Autodesk Inventor part; units mm, degrees
ref_plane "YZ Plane" through (0, 0, 0) normal (1, 0, 0) x (0, 1, 0)
ref_plane "XZ Plane" through (0, 0, 0) normal (0, 1, 0) x (-1, 0, 0)
ref_plane "XY Plane" through (0, 0, 0) normal (0, 0, 1) x (1, 0, 0)
sketch "Sketch1" plane through (0, 0, 0) normal (0, 1, 0) x (-1, 0, 0)
  line L0 (0, 0) -> (711.2, 0)
  line L1 (711.2, 0) -> (711.2, -812.8)
  line L2 (711.2, -812.8) -> (0, -812.8)
  line L3 (0, -812.8) -> (0, 0)
  line L4 (0, 0) -> (711.2, 0)
  line L5 (711.2, 0) -> (711.2, -76.2)
  line L6 (0, -76.2) -> (0, 0)
  line L7 (0, -812.8) -> (711.2, -812.8)
  line L8 (711.2, -812.8) -> (711.2, -736.6)
  line L9 (0, -736.6) -> (0, -812.8)
  line L10 (0, 0) -> (25.4, 0)
  line L11 (25.4, -76.2) -> (25.4, -736.6)
  line L12 (25.4, -812.8) -> (0, -812.8)
  line L13 (0, -812.8) -> (0, 0)
  line L14 (711.2, 0) -> (685.8, 0)
  line L15 (685.8, -76.2) -> (685.8, -736.6)
  line L16 (685.8, -812.8) -> (711.2, -812.8)
  line L17 (711.2, -812.8) -> (711.2, 0)
  line L18 (685.8, -736.6) -> (635, -736.6)
  line L19 (615.95, -736.6) -> (615.95, -76.2)
  line L20 (635, -76.2) -> (635, -736.6)
  line L21 (25.4, -736.6) -> (76.2, -736.6)
  line L22 (95.25, -736.6) -> (95.25, -76.2)
  line L23 (76.2, -76.2) -> (76.2, -736.6)
  line L24 (685.8, -76.2) -> (635, -76.2)
  line L25 (685.8, -736.6) -> (635, -736.6)
  line L26 (615.95, -736.6) -> (95.25, -736.6)
  line L27 (76.2, -736.6) -> (25.4, -736.6)
  line L28 (615.95, -76.2) -> (95.25, -76.2)
  line L29 (76.2, -76.2) -> (25.4, -76.2)
  dimension "d0" = 711.2
  dimension "d1" = 812.8
  dimension "d2" = 76.2
  dimension "d3" = 76.2
  dimension "d4" = 25.4
  dimension "d5" = 25.4
  dimension "d6" = 812.8
  dimension "d10" = 660.4
extrude "Extrusion1" add sketch "Sketch1" along normal blind 3.175
sketch "Sketch2" plane through (0, 3.175, 0) normal (0, 1, 0) x (1, 0, 0)
  line L0 (-711.2, 812.8) -> (0, 812.8)
  line L1 (0, 812.8) -> (0, 0)
  line L2 (0, 0) -> (-711.2, 0)
  line L3 (-711.2, 0) -> (-711.2, 812.8)
  line L4 (-708.025, 809.625) -> (-3.175, 809.625)
  line L5 (-3.175, 809.625) -> (-3.175, 3.175)
  line L6 (-3.175, 3.175) -> (-708.025, 3.175)
  line L7 (-708.025, 3.175) -> (-708.025, 809.625)
extrude "Extrusion2" add sketch "Sketch2" along normal blind 73.025
sketch "Sketch3" plane through (0, 0, 0) normal (0, -1, 0) x (1, 0, 0)
  line L0 (-25.4, -76.2) -> (-25.4, -50.8)
  line L1 (-25.4, -50.8) -> (-685.8, -50.8)
  line L2 (-685.8, -50.8) -> (-685.8, -762)
  line L3 (-685.8, -762) -> (-25.4, -762)
  line L4 (-25.4, -762) -> (-25.4, -50.8)
  line L5 (-25.4, -76.2) -> (-76.2, -76.2)
  line L6 (-76.2, -76.2) -> (-76.2, -50.8)
  line L7 (-95.25, -76.2) -> (-95.25, -50.8)
  line L8 (-95.25, -76.2) -> (-615.95, -76.2)
  line L9 (-615.95, -76.2) -> (-615.95, -50.8)
  line L10 (-635, -76.2) -> (-635, -50.8)
  line L11 (-635, -76.2) -> (-685.8, -76.2)
  line L12 (-95.25, -736.6) -> (-95.25, -762)
  line L13 (-95.25, -736.6) -> (-615.95, -736.6)
  line L14 (-615.95, -736.6) -> (-615.95, -762)
  line L15 (-635, -736.6) -> (-635, -762)
  line L16 (-635, -736.6) -> (-685.8, -736.6)
  line L17 (-635, -50.8) -> (-685.8, -50.8)
  line L18 (-685.8, -50.8) -> (-685.8, -76.2)
  line L19 (-685.8, -736.6) -> (-685.8, -762)
  line L20 (-685.8, -762) -> (-635, -762)
  line L21 (-615.95, -762) -> (-95.25, -762)
  line L22 (-95.25, -762) -> (-95.25, -736.6)
  line L23 (-25.4, -736.6) -> (-25.4, -76.2)
  line L24 (-25.4, -762) -> (-76.2, -762)
  line L25 (-76.2, -762) -> (-76.2, -736.6)
  line L26 (-76.2, -736.6) -> (-25.4, -736.6)
  line L27 (-25.4, -736.6) -> (-25.4, -762)
  point P0 (0, 0)
  dimension "d22" = 25.4
  dimension "d23" = 660.4
  dimension "d24" = 711.2
  dimension "d25" = 25.4
  dimension "d26" = 25.4
extrude "Extrusion3" cut sketch "Sketch3" against normal blind 73.025 contours L5 L6 L1 L0 | L4 L3 L25 L26 | L7 L8 L9 L1 | L3 L14 L13 L12 | L10 L11 L2 L1 | L3 L2 L16 L15
sketch "Sketch4" plane through (-711.2, 0, -812.8) normal (-1, 0, 0) x (0, 0, 1)
  line L0 (812.8, 76.2) -> (406.4, 76.2)
  line L1 (812.8, 76.2) -> (0, 76.2)
  line L2 (762, 0) -> (50.8, 0)
  circle A0 centre (406.4, 63.5) radius 6.35
  circle A1 centre (711.2, 63.5) radius 6.35
  circle A2 centre (101.6, 63.5) radius 6.35
  point P0 (812.8, 0)
  dimension "d29" = 406.4
  dimension "d31" = 12.7
  dimension "d35" = 12.7
  dimension "d36" = 12.7
sketch "Sketch5" plane through (0, 3.175, 0) normal (0, 1, 0) x (1, 0, 0)
  line L0 (-708.025, 3.175) -> (-3.175, 3.175)
  line L1 (-3.175, 809.625) -> (-708.025, 809.625)
  line L2 (-615.95, 3.175) -> (-619.125, 3.175)
  line L3 (-619.125, 3.175) -> (-619.125, 809.625)
  line L4 (-619.125, 809.625) -> (-615.95, 809.625)
  line L5 (-615.95, 809.625) -> (-615.95, 3.175)
  line L6 (-95.25, 809.625) -> (-92.075, 809.625)
  line L7 (-92.075, 809.625) -> (-92.075, 3.175)
  line L8 (-92.075, 3.175) -> (-95.25, 3.175)
  line L9 (-95.25, 3.175) -> (-95.25, 809.625)
  point P0 (0, 0)
  dimension "d37" = 3.175
  dimension "d38" = 3.175
extrude "Extrusion4" add sketch "Sketch5" along normal blind 73.025 contours L3 L1 L5 L0 | L9 L1 L7 L0
extrude "Extrusion5" cut sketch "Sketch4" against normal blind 1016
properties part number "Base"
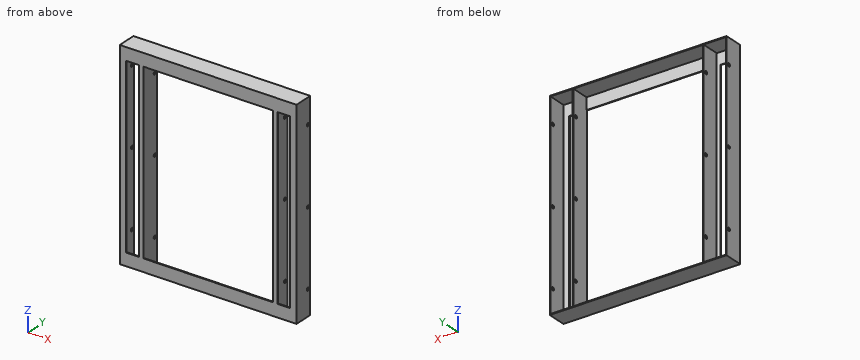
The model under review builds one solid part; all positions refer to its coordinate system, in mm. Round coordinates to 2 decimals unless told otherwise and drop trailing zeros. Write each loop counter-clockwise with the first axis right and the second up, starting at its lowest first coordinate (ties: lowest second). Pieces come first, ordered by that corner, then holes. Notation, with made-up numbers: (-34, 50) - (-1, 50) arc R17 cw to (-1, 73) - close; hole circle Ø7 at (3, -9.5). An arc over 180 degrees is marked (long way). One line per item, written item: value. Start each with the question number.
1. To check wall thickness, follow L1, parallel to X at y = 58, z = -57 (3 decimals); L2, parallel to X at y = 3, z = -294; L3, parallel to Y at x = -94.1, z = -406.4. State the ranges of each line that lie inside material, in increasing order. Write a range as from..to.
2. Consider section A-A on x = -214. Write out the cut boundary in (y, z) (3 decimals), and give its area (3 significant figures).
3. Consider section B-B on z = -142. Write out the cut boundary in (x, y) (3 decimals), and give its area (3 significant figures).
Checks:
1. L1: x = -711.2..-708.025, -619.125..-615.95, -95.25..-92.075, -3.175..0
1. L2: x = -711.2..-685.8, -635..-615.95, -95.25..-76.2, -25.4..0
1. L3: y = 0..57.15, 69.85..76.2
2. outline: (0, -812.8) - (76.2, -812.8) - (76.2, -809.625) - (3.175, -809.625) - (3.175, -762) - (0, -762) - close; (0, -50.8) - (3.175, -50.8) - (3.175, -3.175) - (76.2, -3.175) - (76.2, 0) - (0, 0) - close
2. area: 786 mm^2
3. outline: (-711.2, 0) - (-685.8, 0) - (-685.8, 3.175) - (-708.025, 3.175) - (-708.025, 76.2) - (-711.2, 76.2) - close; (-635, 0) - (-615.95, 0) - (-615.95, 76.2) - (-619.125, 76.2) - (-619.125, 3.175) - (-635, 3.175) - close; (-95.25, 0) - (-76.2, 0) - (-76.2, 3.175) - (-92.075, 3.175) - (-92.075, 76.2) - (-95.25, 76.2) - close; (-25.4, 0) - (0, 0) - (0, 76.2) - (-3.175, 76.2) - (-3.175, 3.175) - (-25.4, 3.175) - close
3. area: 1,210 mm^2
